Check sheet for the modelled part. Datum: model origin and axes. Units: mm. A direction names the side the tool comes from. Round coordinates to 2 decimals unless told otherwise and drop trailing zeros. Loops run counter-clockwise (first coordinate to the right, second up) from the corner with the lowest first, then second, coordinate; pieces in that order, holes last. Notation, with made-up numbers: (34, 28.5) -> (50, 28.5) arc R14 ccw to (50, 34.5) -> close; hole circle Ø11 at (7.25, 85). An arc over 180 degrees is marked (long way). Use one line per item in the form item = value. Start each with the question number.
(1) Sectioned sample at B-B (z = 0). Record the cut outline in (x, y).
(2) Sectioned sample at D-D (y = 9.5). Record the cut outline in (x, z), and give its area (3 significant figures).
(3) Set-up check for faces 1 (the flat face through (-29, -15, -52)), 2 (the flat face through (14, -17, 1)): record each of +Z, -Z, +X, -X, +Y, -Y from which the full face is reachable in a straight line by a thin tool's end or side.
(4) Material ranges on probe 1 along Y at (x, z) = (24.5, 57.5); probe 2 along Z at (x, y) = (0, -0.5), recorded low to high. Write a range as [from, to].
(5) Draft check along Y on faces 3 (the flat face through (-29, 15, 52)), 4 (the flat face through (14, 17, -1)), 5 (the cylindrical face through (62, 16.49, -19.52)). Enter one of: released by +Y, released by -Y, zero draft, split by the parting line, or undercut.
(6) Sectioned sample at C-C (y = 0). Record the cut outline in (x, z).
(7) Sectioned sample at A-A (x = 0). Record the cut outline in (y, z).
(8) Go/stop test with flat-tipped pins: pin 1 (5 mm diameter, centred on y = 13, z = 20, fed in from +X); pin 2 (1.5 mm diameter, centred on y = 6, z = -4, fed in from -X); pin 3 (1.5 mm diameter, centred on x = 26.5, y = -2.5, fed in from -Z). Record where each tip stops, or that it passes through.
from build123d import *

# Parameters (mm, degrees)
SKETCH1_R                = 50
BOSS_EXTRUDE1_DEPTH      = 15
BOSS_EXTRUDE1_DEPTH_BACK = 15
SKETCH2_R                = 65
BOSS_EXTRUDE2_DEPTH      = 2
SKETCH3_R                = 65
BOSS_EXTRUDE3_DEPTH      = 2
FILLET1_R                = 9
FILLET2_R                = 1
FILLET3_R                = 1
FILLET4_R                = 9
CUT_EXTRUDE1_REACH       = 36
SKETCH4_R                = 10


with BuildPart() as part:
    # Sketch1 → Boss-Extrude1 (new body, two sides)
    with BuildSketch(Plane(origin=(0, 0, 0), x_dir=(1, 0, 0), z_dir=(0, 1, 0))) as boss_extrude1_sk:
        Circle(SKETCH1_R)
    extrude(amount=BOSS_EXTRUDE1_DEPTH)
    extrude(boss_extrude1_sk.sketch, amount=-BOSS_EXTRUDE1_DEPTH_BACK)

    # Sketch2 → Boss-Extrude2 (add)
    with BuildSketch(Plane.XZ.offset(15)):
        Circle(SKETCH2_R)
    extrude(amount=BOSS_EXTRUDE2_DEPTH)

    # Sketch3 → Boss-Extrude3 (add)
    with BuildSketch(Plane(origin=(0, 15, 0), x_dir=(1, 0, 0), z_dir=(0, 1, 0))):
        Circle(SKETCH3_R)
    extrude(amount=BOSS_EXTRUDE3_DEPTH)

    # Fillet1
    fillet1_edges = [part.edges().sort_by_distance(p)[0] for p in [
        (-50, -15, 0),
    ]]
    fillet(fillet1_edges, radius=FILLET1_R)

    # Fillet2
    fillet2_edges = [part.edges().sort_by_distance(p)[0] for p in [
        (-65, -15, 0),
    ]]
    fillet(fillet2_edges, radius=FILLET2_R)

    # Fillet3
    fillet3_edges = [part.edges().sort_by_distance(p)[0] for p in [
        (-65, 15, 0),
    ]]
    fillet(fillet3_edges, radius=FILLET3_R)

    # Fillet4
    fillet4_edges = [part.edges().sort_by_distance(p)[0] for p in [
        (-50, 15, 0),
    ]]
    fillet(fillet4_edges, radius=FILLET4_R)

    # Sketch4 → Cut-Extrude1 (cut, up to next)
    with BuildSketch(Plane(origin=(0, 17, 0), x_dir=(1, 0, 0), z_dir=(0, 1, 0)), mode=Mode.PRIVATE) as cut_extrude1_sk1:
        Circle(SKETCH4_R)
    cut_extrude1_tool1 = extrude(cut_extrude1_sk1.sketch, amount=-CUT_EXTRUDE1_REACH, mode=Mode.PRIVATE) & part.part
    add(cut_extrude1_tool1.solids().sort_by_distance((0, 17, 0))[0], mode=Mode.SUBTRACT)


solid = part.part
Checks:
q1.outline = (-65, -17) -> (-10, -17) -> (-10, 17) -> (-65, 17) -> (-65, 16) arc R1 ccw to (-64, 15) -> (-59, 15) arc R9 cw to (-50, 6) -> (-50, -6) arc R9 cw to (-59, -15) -> (-64, -15) arc R1 ccw to (-65, -16) -> close; (10, -17) -> (65, -17) -> (65, -16) arc R1 ccw to (64, -15) -> (59, -15) arc R9 cw to (50, -6) -> (50, 6) arc R9 cw to (59, 15) -> (64, 15) arc R1 ccw to (65, 16) -> (65, 17) -> (10, 17) -> close
q2.outline = circle Ø101.42 at (0, 0); hole circle Ø20 at (0, 0)
q2.area = 7,760 mm2
q3.face_1 = none
q3.face_2 = +Z, -Z, +X, -X, -Y
q4.probe_1 = [-17, -15], [15, 17]
q4.probe_2 = [-50, -10], [10, 50]
q5.face_3 = undercut
q5.face_4 = released by +Y
q5.face_5 = zero draft
q6.outline = circle Ø100 at (0, 0); hole circle Ø20 at (0, 0)
q7.outline = (-17, -65) -> (-16, -65) arc R1 ccw to (-15, -64) -> (-15, -59) arc R9 cw to (-6, -50) -> (6, -50) arc R9 cw to (15, -59) -> (15, -64) arc R1 ccw to (16, -65) -> (17, -65) -> (17, -10) -> (-17, -10) -> close; (-17, 10) -> (17, 10) -> (17, 65) -> (16, 65) arc R1 ccw to (15, 64) -> (15, 59) arc R9 cw to (6, 50) -> (-6, 50) arc R9 cw to (-15, 59) -> (-15, 64) arc R1 ccw to (-16, 65) -> (-17, 65) -> close
q8.pin_1 = 61.86
q8.pin_2 = -49.9
q8.pin_3 = -42.86
